Could you check a few things on this model? Use its own coordinates, in mm. Face numbers are marked on the shaded views. A direction names the side the tool comes from. Coordinates: 2 decimals unless noted, no trailing zeros. Loops run counter-clockwise (first coordinate to the right, second up) from the corner with the lowest first, then second, coordinate; pieces in that order, holes last.
1) For the marked faces 1 and 2, which set-ups out of +Z, -Z, +X, -X, +Y, -Y let a thin tool reach every point of the face, with its end or its side?
2) If I drill on line 1 along Z through (x, y) = (0.5, 43.5); line 2 along Y through (x, z) = (20, 7.5); line 3 along X through (y, z) = (13.5, 2.5), over which ranges is the centre line in solid material (lowest first)?
3) Imagine slicing it at A-A on y = 50.5. Please give me the cut outline in (x, z).
4) Will these pins go through, and if not, where does the flat tip stop? P1, Ø3, axis at y = 52.5, z = 17.5, coming from the -X side; P2, Ø12, axis at x = -16, z = -11, coming from the +Y side; P3, Ø2, axis at y = 32, z = 18.5, coming from the -X side; P4, Ø6, axis at x = 9, y = 22, coming from the +Z side.
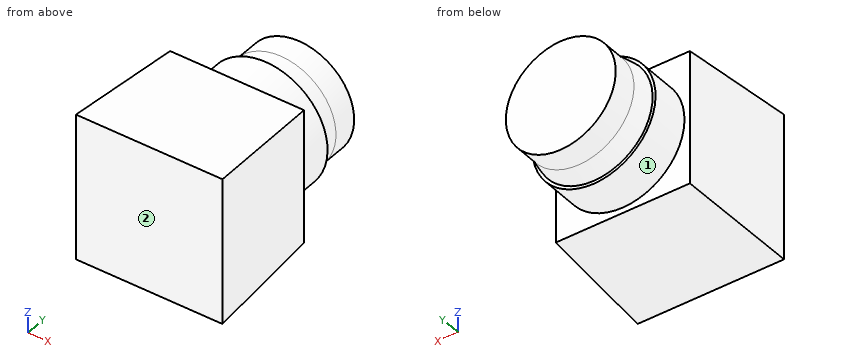
```python
from build123d import *

# Parameters (mm, degrees)
ESBO_O1_W                = 50
ESBO_O1_H                = 50
RESSALTO_EXTRUS_O1_DEPTH = 41
RESSALTO_EXTRUS_O1_TAPER = 3


with BuildPart() as part:
    # Esboço1 → Ressalto-extrusão1 (new body)
    with BuildSketch(Plane(origin=(0, 0, 0), x_dir=(1, 0, 0), z_dir=(0, 1, 0))):
        Rectangle(ESBO_O1_W, ESBO_O1_H)
    extrude(amount=RESSALTO_EXTRUS_O1_DEPTH, taper=RESSALTO_EXTRUS_O1_TAPER)

    # Esboço2 → Revolução1 (revolve)
    with BuildSketch(Plane(origin=(0, 0, 0), x_dir=(0, 0, -1), z_dir=(1, 0, 0))):
        Polygon((0, 41), (0, 70), (18.75, 70), (18.75, 61.5), (20, 54.5), (21, 54.5), (21, 41), align=None)
    revolve(axis=Axis((0, 41, 0), (0, 1, 0)))


solid = part.part
```
Filled in:
1. face 1: +Y
1. face 2: +Z, -Z, +X, -X, -Y
2. line 1: z = -20.99 to 20.99
2. line 2: y = 0 to 41
2. line 3: x = -24.29 to 24.29
3. outline: circle Ø42 at (0, 0)
4. P1: stops at x = -13.6
4. P2: stops at y = 70
4. P3: stops at x = -23.38
4. P4: stops at z = 24
